Model file for the job. Use its own axes, mm. Face numbers are marked on the shaded views. A direction names the side the tool comes from. Coordinates: 2 decimals unless noted, no trailing zeros. Loops run counter-clockwise (first coordinate to the right, second up) from the corner with the lowest first, then second, coordinate; pieces in that order, holes last. Notation, with made-up numbers: M -39.75,10 L -19.75,10 A18 ccw -19.75,29 Z; hole C -23,-12.5 d6. An arc over 180 degrees is marked long. Write item = value, one per line. Start each with the question number.
from build123d import *

# Parameters (mm, degrees)
BOSS_EXTRU_1_DEPTH                = 5
DIAM_TRE_DU_PER_AGE_2_0_2_1_D     = 2
DIAM_TRE_DU_PER_AGE_2_0_2_1_DEPTH = 10
DIAM_TRE_DU_PER_AGE_2_0_2_1_TIP   = 0.600860619
CHANFREIN1_SIZE                   = 0.4


with BuildPart() as part:
    # Esquisse1 → Boss.-Extru.1 (new body)
    with BuildSketch(Plane(origin=(0, 0, 0), x_dir=(0, -1, 0), z_dir=(-1, 0, 0))):
        Polygon((-1.443375672, -2.5), (1.443375674, -2.5), (2.886751347, 1e-09), (1.443375673, 2.5), (-1.443375673, 2.5), (-2.886751345, 1e-09), align=None)
    extrude(amount=-BOSS_EXTRU_1_DEPTH)

    # Esquisse2 → Révolution1 (revolve)
    with BuildSketch(Plane(origin=(0, 0, 0), x_dir=(-1, 0, 0), z_dir=(0, 0, -1)), mode=Mode.PRIVATE) as r_volution1_sk:
        Polygon((0, 1.157712139), (0, 0.13332547), (5, 0.13332547), (5, 1.63332547), (1.215350333, 1.63332547), (1.215350333, 1.157712139), align=None)
    revolve(r_volution1_sk.sketch.rotate(Axis((0, 0.13332547, 0), (-1, 0, 0)), 270), axis=Axis((0, 0.13332547, 0), (-1, 0, 0)))

    # Diamètre du perçage Ø2.0 (2)1
    with Locations(Plane(origin=(5, 0, 0), x_dir=(0, 0, -1), z_dir=(1, 0, 0))):
        with Locations((0.015228416, -0.068295067)):
            Hole(DIAM_TRE_DU_PER_AGE_2_0_2_1_D / 2, depth=DIAM_TRE_DU_PER_AGE_2_0_2_1_DEPTH)
            with Locations((0, 0, -(DIAM_TRE_DU_PER_AGE_2_0_2_1_DEPTH + DIAM_TRE_DU_PER_AGE_2_0_2_1_TIP / 2))):  # 118° drill point
                Cone(0, DIAM_TRE_DU_PER_AGE_2_0_2_1_D / 2, DIAM_TRE_DU_PER_AGE_2_0_2_1_TIP, mode=Mode.SUBTRACT)

    # Chanfrein1
    # the kernel refuses this chamfer: 0.4 mm, written as the material it takes off along each edge
    with BuildSketch(Plane(origin=(-5, 0.13332547, 0), x_dir=(0, 0, 1), z_dir=(0, -1, 0))) as chanfrein1_piece_1:
        Polygon((1.5, -CHANFREIN1_SIZE), (1.5 - CHANFREIN1_SIZE, 0), (1.5, 0), align=None)
    revolve(axis=Axis((-5, 0.13332547, 0), (-1, 0, 0)), mode=Mode.SUBTRACT)


solid = part.part
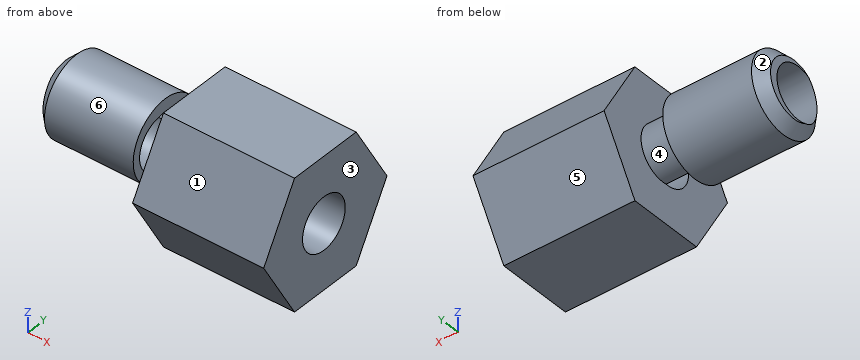
Item 1: Cut at D-D (y = 1.95). Give the cut face in (x, z).
Item 2: Probe L1, parallel to Y at x = -3.25, z = 0; L2, parallel to X at y = -0.9, z = 1.55; L3, parallel to Z at x = 2.5, y = -0.45. List the from-to ranges inside material, lowest first.
Item 3: Cut at A-A (z = -0.7). Give the number of separate pieces and of enclosed holes in the cut face, plus the area to 3 significant figures.
Item 4: Pin check, flat tips, straight feed: pin 1 Ø2 at (x, z) = (-0.5, -1.5) entering from -Y; pin 2 Ø1 at (x, y) = (3.5, 2.5) entering from +Z; pin 3 Ø1.5 at (x, z) = (-2.5, -0.5) entering from +Y. Stop position of each tip, or through.
Item 5: Cut at B-B (y = -2). Give the cut face in (x, z).
Item 6: Pull direction X, two halves, no side cores. Call the marked faces 1, 2, 3 and 4: +X half, -X half, draft (parallel to the pull), parting line (faces both ways), or undercut.
Item 7: 3-axis set-ups, long thin cutter, end or side, ignore diameter. For the marked faces 5 and 6: which of +Z, -Z, +X, -X, +Y, -Y reach the whole face in a straight line?
Reported:
q1.outline = M 0,-1.62 L 5,-1.62 L 5,1.62 L 0,1.62 Z
q2.L1 = -1.37 to -1.07, 0.93 to 1.63
q2.L2 = 0 to 5
q2.L3 = -2.5 to -0.94, 0.91 to 2.5
q3.separate_pieces = 3
q3.enclosed_holes = 0
q3.area = 22.1 mm^2
q4.pin_1 = -2.52
q4.pin_2 = 1.54
q4.pin_3 = 1.63
q5.outline = M 0,-1.54 L 5,-1.54 L 5,1.54 L 0,1.54 Z
q6.face_1 = draft
q6.face_2 = -X half
q6.face_3 = +X half
q6.face_4 = undercut
q7.face_5 = -Z, +X, -X, +Y
q7.face_6 = -X
